```python
from build123d import *

# Parameters (mm, degrees)
BOX001_W      = 1
BOX001_H      = 5
BOX001_DEPTH  = 12
ARRAY_X_COUNT = 6
ARRAY_X_PITCH = 28
BOX_W         = 150
BOX_H         = 5
BOX_DEPTH     = 20


with BuildPart() as array:
    # Box001 → Box001 (new body)
    with BuildSketch(Plane.XY):
        with Locations((0.5, 2.5)):
            Rectangle(BOX001_W, BOX001_H)
    extrude(amount=BOX001_DEPTH)

    # Array X: Array ×6


with BuildPart() as array_1:
    add(array.part)
    with Locations(*[(i * ARRAY_X_PITCH, 0, 0) for i in range(1, ARRAY_X_COUNT)]):
        add(array.part)


with BuildPart() as cut:
    # Box → Box (new body)
    with BuildSketch(Plane(origin=(-5, 0, 0), x_dir=(1, 0, 0), z_dir=(0, 0, 1))):
        with Locations((75, 2.5)):
            Rectangle(BOX_W, BOX_H)
    extrude(amount=BOX_DEPTH)

    # Cut: cut Array
    add(array_1.part, mode=Mode.SUBTRACT)


solid = cut.part
```
For this review, take the finished solid that the model builds, in its own axes (mm). A direction names the side the tool comes from. Round coordinates to 2 decimals unless told otherwise and drop trailing zeros. Loops run counter-clockwise (first coordinate to the right, second up) from the corner with the lowest first, then second, coordinate; pieces in that order, holes last.
Q1. Mouldability with a two-part tool opening along X and no side actions: class faces 3 (the face through (-5, 2, 10)), 4 (the face through (112, 2, 6)), 5 (the face through (69, 0, 10)) as +X half, -X half, draft (parallel to the pull), parting line (faces both ways), or undercut.
Result sheet:
face 3: -X half
face 4: undercut
face 5: draft
Q2. Machinability: for faces 1 (the face through (0, 2, 6)), 2 (the face through (69, 5, 10)), which of the approach directions +Z, -Z, +X, -X, +Y, -Y give a long, thin tool a straight path to every point of the face, cutting with its end or side? Answer none if there is none.
Result sheet:
face 1: -Z, +Y, -Y
face 2: +Z, -Z, +X, -X, +Y
Q3. Add section A-A on z = 8.25. Write out the cut boundary in (x, y).
Result sheet:
outline: (-5, 0) - (0, 0) - (0, 5) - (-5, 5) - close; (1, 0) - (28, 0) - (28, 5) - (1, 5) - close; (29, 0) - (56, 0) - (56, 5) - (29, 5) - close; (57, 0) - (84, 0) - (84, 5) - (57, 5) - close; (85, 0) - (112, 0) - (112, 5) - (85, 5) - close; (113, 0) - (140, 0) - (140, 5) - (113, 5) - close; (141, 0) - (145, 0) - (145, 5) - (141, 5) - close
Q4. Add section B-B on y = 1.25. Write out the cut boundary in (x, z), plus the area to 3 significant figures.
Result sheet:
outline: (-5, 0) - (0, 0) - (0, 12) - (1, 12) - (1, 0) - (28, 0) - (28, 12) - (29, 12) - (29, 0) - (56, 0) - (56, 12) - (57, 12) - (57, 0) - (84, 0) - (84, 12) - (85, 12) - (85, 0) - (112, 0) - (112, 12) - (113, 12) - (113, 0) - (140, 0) - (140, 12) - (141, 12) - (141, 0) - (145, 0) - (145, 20) - (-5, 20) - close
area: 2,930 mm2
Q5. Insertion check: pin 1 Ø0.8 at (x, y) = (0.5, 3.5) entering from -Z; pin 2 Ø1.1 at (x, y) = (56.5, 3.5) entering from -Z. Each pin has a flat end and moves straight along its axis. Give the tip position at first contact, or say it passes through.
Result sheet:
pin 1: stops at z = 12
pin 2: stops at z = 0
